Build history of the part. All positions in model axes, mm. A direction names the side the tool comes from. Coordinates: 2 decimals unless noted, no trailing zeros. Write each loop counter-clockwise with the first axis right and the second up, starting at its lowest first coordinate (ties: lowest second). Pieces come first, ordered by that corner, then holes.
```python
from build123d import *

# Parameters (mm, degrees)
SKETCH1_R                = 150
BOSS_EXTRUDE1_DEPTH      = 75
CHAMFER1_SIZE            = 10
BOSS_EXTRUDE2_START      = -10
BOSS_EXTRUDE2_DEPTH      = 10
CHAMFER2_SIZE            = 10
BOSS_EXTRUDE3_DEPTH      = 10
BOSS_EXTRUDE4_DEPTH      = 3.5
CIRPATTERN1_COUNT        = 4
CIRPATTERN1_COPY_1_DEPTH = 10
CIRPATTERN1_COPY_2_DEPTH = 10
CIRPATTERN1_COPY_3_DEPTH = 10
CIRPATTERN1_COPY_4_DEPTH = 3.5
CIRPATTERN1_COPY_5_DEPTH = 3.5
CIRPATTERN1_COPY_6_DEPTH = 3.5
CUT_EXTRUDE1_DEPTH       = 60
SKETCH6_R                = 110
BOSS_EXTRUDE5_DEPTH      = 10
CHAMFER3_SIZE            = 15
SKETCH7_R                = 15
BOSS_EXTRUDE6_DEPTH      = 20


with BuildPart() as part:
    # Sketch1 → Boss-Extrude1 (new body)
    with BuildSketch(Plane(origin=(0, 0, 0), x_dir=(0, 1, 0), z_dir=(0, 0, 1))):
        with Locations(Location((0, 0, 0), (0, 0, 270))):
            Circle(SKETCH1_R)
    extrude(amount=BOSS_EXTRUDE1_DEPTH)

    # Chamfer1
    chamfer1_edges = [part.edges().sort_by_distance(p)[0] for p in [
        (-150, 0, 0),
    ]]
    chamfer(chamfer1_edges, length=CHAMFER1_SIZE)

    # Sketch2 → Boss-Extrude2 (add)
    with BuildSketch(Plane.XY.offset(75).offset(BOSS_EXTRUDE2_START)):
        with BuildLine():
            Line((-200, 37.5), (-200, -37.5))
            Line((-200, -37.5), (-145.236875483, -37.5))
            ThreePointArc((-145.236875483, -37.5), (-150, 0), (-145.236875483, 37.5))
            Line((-145.236875483, 37.5), (-200, 37.5))
        make_face()
    boss_extrude2 = extrude(amount=BOSS_EXTRUDE2_DEPTH)

    # Chamfer2
    chamfer2_edges = [part.edges().sort_by_distance(p)[0] for p in [
        (-200, 37.5, 70),
        (-200, -37.5, 70),
    ]]
    chamfer(chamfer2_edges, length=CHAMFER2_SIZE)

    # Sketch3 → Boss-Extrude3 (add)
    with BuildSketch(Plane(origin=(0, 37.5, 0), x_dir=(-1, 0, 0), z_dir=(0, 1, 0))):
        Polygon((145.236875483, 65), (145.236875483, 9.354005049), (172.32, 9.354005049), (190, 65), align=None)
    boss_extrude3 = extrude(amount=-BOSS_EXTRUDE3_DEPTH)

    # Sketch4 → Boss-Extrude4 (add)
    with BuildSketch(Plane(origin=(0, 0, 65), x_dir=(1, 0, 0), z_dir=(0, 0, -1))):
        Polygon((-190, -9.409610349), (-195.196152423, -12.409610349), (-195.196152423, -18.409610349), (-190, -21.409610349), (-184.803847577, -18.409610349), (-184.803847577, -12.409610349), align=None)
    boss_extrude4 = extrude(amount=BOSS_EXTRUDE4_DEPTH)

    # Mirror1: Boss-Extrude3, Boss-Extrude4 across plane
    add(boss_extrude3.mirror(Plane.ZX))
    add(boss_extrude4.mirror(Plane.ZX))

    # CirPattern1: Boss-Extrude2, Boss-Extrude3, Boss-Extrude4 ×4 about axis
    cirpattern1_axis = Axis((0, 0, 0), (0, 0, 1))
    add([boss_extrude2.rotate(cirpattern1_axis, i * 360 / CIRPATTERN1_COUNT) for i in range(1, CIRPATTERN1_COUNT)])
    add([boss_extrude3.rotate(cirpattern1_axis, i * 360 / CIRPATTERN1_COUNT) for i in range(1, CIRPATTERN1_COUNT)])
    add([boss_extrude4.rotate(cirpattern1_axis, i * 360 / CIRPATTERN1_COUNT) for i in range(1, CIRPATTERN1_COUNT)])

    # CirPattern1 copy 1 sketch → CirPattern1 copy 1 (add)
    with BuildSketch(Plane(origin=(37.5, 0, 0), x_dir=(0, -1, 0), z_dir=(1, 0, 0))):
        Polygon((145.236875483, -65), (145.236875483, -9.354005049), (172.32, -9.354005049), (190, -65), align=None)
    extrude(amount=-CIRPATTERN1_COPY_1_DEPTH)

    # CirPattern1 copy 2 sketch → CirPattern1 copy 2 (add)
    with BuildSketch(Plane(origin=(0, 37.5, 0), x_dir=(1, 0, 0), z_dir=(0, 1, 0))):
        Polygon((145.236875483, -65), (145.236875483, -9.354005049), (172.32, -9.354005049), (190, -65), align=None)
    extrude(amount=-CIRPATTERN1_COPY_2_DEPTH)

    # CirPattern1 copy 3 sketch → CirPattern1 copy 3 (add)
    with BuildSketch(Plane(origin=(-37.5, 0, 0), x_dir=(0, 1, 0), z_dir=(-1, 0, 0))):
        Polygon((145.236875483, -65), (145.236875483, -9.354005049), (172.32, -9.354005049), (190, -65), align=None)
    extrude(amount=-CIRPATTERN1_COPY_3_DEPTH)

    # CirPattern1 copy 4 sketch → CirPattern1 copy 4 (add)
    with BuildSketch(Plane.YX.offset(-65)):
        Polygon((-190, 9.409610349), (-195.196152423, 12.409610349), (-195.196152423, 18.409610349), (-190, 21.409610349), (-184.803847577, 18.409610349), (-184.803847577, 12.409610349), align=None)
    extrude(amount=CIRPATTERN1_COPY_4_DEPTH)

    # CirPattern1 copy 5 sketch → CirPattern1 copy 5 (add)
    with BuildSketch(Plane(origin=(0, 0, 65), x_dir=(-1, 0, 0), z_dir=(0, 0, -1))):
        Polygon((-190, 9.409610349), (-195.196152423, 12.409610349), (-195.196152423, 18.409610349), (-190, 21.409610349), (-184.803847577, 18.409610349), (-184.803847577, 12.409610349), align=None)
    extrude(amount=CIRPATTERN1_COPY_5_DEPTH)

    # CirPattern1 copy 6 sketch → CirPattern1 copy 6 (add)
    with BuildSketch(Plane(origin=(0, 0, 65), x_dir=(0, -1, 0), z_dir=(0, 0, -1))):
        Polygon((-190, 9.409610349), (-195.196152423, 12.409610349), (-195.196152423, 18.409610349), (-190, 21.409610349), (-184.803847577, 18.409610349), (-184.803847577, 12.409610349), align=None)
    extrude(amount=CIRPATTERN1_COPY_6_DEPTH)

    # Sketch5 → Cut-Extrude1 (cut)
    with BuildSketch(Plane(origin=(0, 0, 0), x_dir=(1, 0, 0), z_dir=(0, 0, -1))):
        with BuildLine():
            Line((-112.583302492, -65), (-129.903810568, -75))
            ThreePointArc((-129.903810568, -75), (-106.066017178, -106.066017178), (-75, -129.903810568))
            Line((-75, -129.903810568), (-65, -112.583302492))
            ThreePointArc((-65, -112.583302492), (-91.923881554, -91.923881554), (-112.583302492, -65))
        make_face()
    extrude(amount=-CUT_EXTRUDE1_DEPTH, mode=Mode.SUBTRACT)

    # Sketch6 → Boss-Extrude5 (add)
    with BuildSketch(Plane(origin=(0, 0, 0), x_dir=(1, 0, 0), z_dir=(0, 0, -1))):
        with Locations(Location((0, 0, 0), (0, 0, 180))):
            Circle(SKETCH6_R)
    extrude(amount=BOSS_EXTRUDE5_DEPTH)

    # Chamfer3
    # the kernel refuses this chamfer: 15 mm, written as the material it takes off along each edge
    with BuildSketch(Plane(origin=(0, 0, -10), x_dir=(-1, 0, 0), z_dir=(0, -1, 0))) as chamfer3_piece_1_section:
        Polygon((110, -CHAMFER3_SIZE), (110 - CHAMFER3_SIZE, 0), (110, 0), align=None)
    chamfer3_piece_1 = revolve(axis=Axis((0, 0, -10), (0, 0, -1)), mode=Mode.PRIVATE)
    chamfer3_piece_1 = split(chamfer3_piece_1, bisect_by=Plane(origin=(100.081022807, 0, 0), z_dir=(0, 0, -1)), keep=Keep.TOP, mode=Mode.PRIVATE)
    add(chamfer3_piece_1, mode=Mode.SUBTRACT)

    # Sketch7 → Boss-Extrude6 (add)
    with BuildSketch(Plane(origin=(0, 0, -10), x_dir=(1, 0, 0), z_dir=(0, 0, -1))):
        with Locations(Location((0, 0, 0), (0, 0, 180))):
            Circle(SKETCH7_R)
    extrude(amount=BOSS_EXTRUDE6_DEPTH)


solid = part.part
```
1. Probe line 1 along Y through (x, z) = (-155, 29); line 2 along Z through (x, y) = (-182, -16). List the from-to ranges inside material, lowest first.
Computed values:
line 1: y = -37.5 to -27.5, 27.5 to 37.5
line 2: z = 65 to 75
2. 3-axis set-ups, long thin cutter, end or side, ignore diameter. For faces 1 (the face through (-15, -190, 61.5)), 2 (the face through (-91.586, 92.26, 29.58)), 3 (the face through (0, 0, -30)), 4 (the face through (-190, 15, 61.5)), 5 (the face through (167, 37.5, 42)): which of +Z, -Z, +X, -X, +Y, -Y reach the whole face in a straight line?
Computed values:
face 1: -Z, -Y
face 2: -Z
face 3: -Z, +X, -X, +Y, -Y
face 4: -Z, -X
face 5: +Z, -Z, +X, +Y
3. Flat gauge pins, fed straight in: pin 1 (5 mm diameter, centred on x = -43.5, z = 11.5, fed in from +Y); pin 2 (5 mm diameter, centred on x = 131.5, y = 77, fed in from -Z); pin 3 (3 mm diameter, centred on x = -17, z = 17.5, fed in from +Y); pin 4 (2 mm diameter, centred on y = 104.5, z = -4.5, fed in from +X). Where does each tip first touch, or does it go through?
Computed values:
pin 1: stops at y = 144.29
pin 2: stops at z = 9.89
pin 3: stops at y = 149.2
pin 4: passes through
4. Mould opens along Y. For faces 6 (the face through (-162, -37.5, 43)), 7 (the face through (163, -27.5, 38)), 8 (the face through (37.5, 166, 42)) say: +Y half, -Y half, draft (parallel to the pull), parting line (faces both ways), or undercut.
Computed values:
face 6: -Y half
face 7: undercut
face 8: draft
5. Saw through at A-A on y = 0. List the corners of the cut face in (x, z), plus the area to 3 significant figures.
Computed values:
outline: (-200, 65) - (-150, 65) - (-150, 10) - (-140, 0) - (-105, 0) - (-95, -10) - (-15, -10) - (-15, -30) - (15, -30) - (15, -10) - (95, -10) - (105, 0) - (140, 0) - (150, 10) - (150, 65) - (200, 65) - (200, 75) - (-200, 75) - close
area: 26,000 mm2
